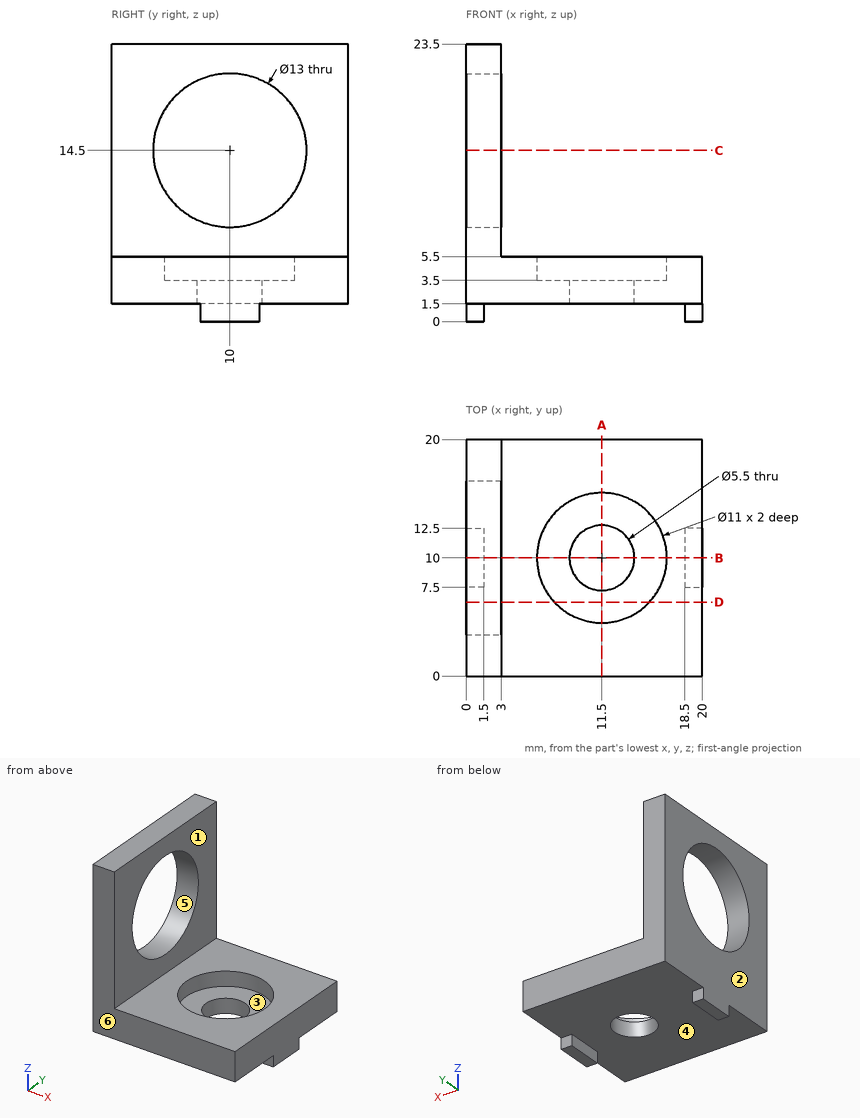
Print and shaded views of the part. All mm, measured from the part's lowest x, y and z. A direction names the side the tool comes from. Coordinates: 2 decimals unless noted, no trailing zeros. Write each loop counter-clockwise with the first axis right and the second up, starting at its lowest first coordinate (ties: lowest second). Pieces come first, ordered by that corner, then holes.
(1) Flat gauge pins, fed straight in: pin 1 (0.8 mm diameter, centred on x = 1, z = 0.5, fed in from -Y); pin 2 (10 mm diameter, centred on x = 9, y = 11, fed in from +Z); pin 3 (5 mm diameter, centred on y = 15.5, z = 10, fed in from -X); pin 4 (1 mm diameter, centred on x = 8.5, y = 2.5, fed in from -Z). Where does each tip first touch, or does it go through?
(2) Cut at C-C, the plane z = 14.5. List the corners of the cut face in (x, y), and give its area (3 significant figures).
(3) Cut at A-A, the plane x = 11.5. List the corners of the cut face in (y, z), and give its area (3 significant figures).
(4) 3-axis set-ups, long thin cutter, end or side, ignore diameter. For the marked faces 1, 2 and 3: which of +Z, -Z, +X, -X, +Y, -Y reach the whole face in a straight line?
(5) Drill centre lines: probe 1 along Y at (x, z) = (11.5, 4.75); probe 2 along Y at (x, z) = (11.5, 2.25); probe 3 along X at (y, z) = (10, 4.5). Where is each one in solid material? Low to high.
(6) Two-plate mould, pull along Y, no slides. Class the marked faces 4, 5 and 6: +Y half, -Y half, draft (parallel to the pull), parting line (faces both ways), or undercut.
(7) Cut at B-B, the plane y = 10. List the corners of the cut face in (x, z).
(8) Cut at D-D, the plane y = 6.25. List the corners of the cut face in (x, z).
Geometry says:
1. pin 1: stops at y = 7.5
1. pin 2: stops at z = 5.5
1. pin 3: stops at x = 0
1. pin 4: stops at z = 1.5
2. outline: (0, 0) - (3, 0) - (3, 3.5) - (0, 3.5) - close; (0, 16.5) - (3, 16.5) - (3, 20) - (0, 20) - close
2. area: 21.0 mm2
3. outline: (0, 1.5) - (7.25, 1.5) - (7.25, 3.5) - (4.5, 3.5) - (4.5, 5.5) - (0, 5.5) - close; (12.75, 1.5) - (20, 1.5) - (20, 5.5) - (15.5, 5.5) - (15.5, 3.5) - (12.75, 3.5) - close
3. area: 47.0 mm2
4. face 1: +Z, +X, +Y, -Y
4. face 2: +Z, -Z, -X, +Y, -Y
4. face 3: +Z
5. probe 1: y = 0 to 4.5, 15.5 to 20
5. probe 2: y = 0 to 7.25, 12.75 to 20
5. probe 3: x = 0 to 6, 17 to 20
6. face 4: draft
6. face 5: undercut
6. face 6: -Y half
7. outline: (0, 0) - (1.5, 0) - (1.5, 1.5) - (8.75, 1.5) - (8.75, 3.5) - (6, 3.5) - (6, 5.5) - (3, 5.5) - (3, 8) - (0, 8) - close; (0, 21) - (3, 21) - (3, 23.5) - (0, 23.5) - close; (14.25, 1.5) - (18.5, 1.5) - (18.5, 0) - (20, 0) - (20, 5.5) - (17, 5.5) - (17, 3.5) - (14.25, 3.5) - close
8. outline: (0, 1.5) - (20, 1.5) - (20, 5.5) - (15.52, 5.5) - (15.52, 3.5) - (7.48, 3.5) - (7.48, 5.5) - (3, 5.5) - (3, 9.19) - (0, 9.19) - close; (0, 19.81) - (3, 19.81) - (3, 23.5) - (0, 23.5) - close
